```python
from build123d import *

# Parameters (mm, degrees)
SKETCH1_R           = 2.25
SKETCH1_W           = 40.1
SKETCH1_H           = 20.1
BOSS_EXTRUDE1_DEPTH = 3.175
FILLET1_R           = 80
FILLET2_R           = 8


with BuildPart() as part:
    # Sketch1 → Boss-Extrude1 (new body)
    with BuildSketch(Plane(origin=(0, 0, 0), x_dir=(1, 0, 0), z_dir=(0, 1, 0))):
        with BuildLine():
            Line((-70, 14), (-40, 14))
            Line((-40, 14), (-39.816062711, 70))
            Line((-39.816062711, 70), (-73.623466631, 79.058666579))
            ThreePointArc((-73.623466631, 79.058666579), (-83.522961568, 96.205094778), (-66.376533369, 106.104589715))
            Line((-66.376533369, 106.104589715), (0, 88.319051202))
            Line((0, 88.319051202), (66.376533369, 106.104589715))
            ThreePointArc((66.376533369, 106.104589715), (83.522961568, 96.205094778), (73.623466631, 79.058666579))
            Line((73.623466631, 79.058666579), (39.816062711, 70))
            Line((39.816062711, 70), (40, 14))
            Line((40, 14), (70, 14))
            ThreePointArc((70, 14), (84, 0), (70, -14))
            Line((70, -14), (40, -14))
            Line((40, -14), (39.816062711, -70))
            Line((39.816062711, -70), (73.623466631, -79.058666579))
            ThreePointArc((73.623466631, -79.058666579), (83.522961568, -96.205094778), (66.376533369, -106.104589715))
            Line((66.376533369, -106.104589715), (0, -88.319051202))
            Line((0, -88.319051202), (-66.376533369, -106.104589715))
            ThreePointArc((-66.376533369, -106.104589715), (-83.522961568, -96.205094778), (-73.623466631, -79.058666579))
            Line((-73.623466631, -79.058666579), (-39.816062711, -70))
            Line((-39.816062711, -70), (-40, -14))
            Line((-40, -14), (-70, -14))
            ThreePointArc((-70, -14), (-84, 0), (-70, 14))
        make_face()
        with Locations(Location((-76.433311385, 99.481809639, 0), (0, 0, 270))):
            Circle(SKETCH1_R, mode=Mode.SUBTRACT)
        with Locations(Location((-79.021501836, 89.822551376, 0), (0, 0, 270))):
            Circle(SKETCH1_R, mode=Mode.SUBTRACT)
        with Locations(Location((-78, 5, 0), (0, 0, 270))):
            Circle(SKETCH1_R, mode=Mode.SUBTRACT)
        with Locations(Location((-79.021501836, -89.822551376, 0), (0, 0, 90))):
            Circle(SKETCH1_R, mode=Mode.SUBTRACT)
        with Locations(Location((-76.433311385, -99.481809639, 0), (0, 0, 90))):
            Circle(SKETCH1_R, mode=Mode.SUBTRACT)
        with Locations(Location((-78, -5, 0), (0, 0, 270))):
            Circle(SKETCH1_R, mode=Mode.SUBTRACT)
        with Locations(Location((78, -5, 0), (0, 0, 90))):
            Circle(SKETCH1_R, mode=Mode.SUBTRACT)
        with Locations(Location((76.433311385, -99.481809639, 0), (0, 0, 270))):
            Circle(SKETCH1_R, mode=Mode.SUBTRACT)
        with Locations(Location((79.021501836, -89.822551376, 0), (0, 0, 270))):
            Circle(SKETCH1_R, mode=Mode.SUBTRACT)
        with Locations(Location((78, 5, 0), (0, 0, 90))):
            Circle(SKETCH1_R, mode=Mode.SUBTRACT)
        with Locations(Location((79.021501836, 89.822551376, 0), (0, 0, 90))):
            Circle(SKETCH1_R, mode=Mode.SUBTRACT)
        with Locations(Location((76.433311385, 99.481809639, 0), (0, 0, 90))):
            Circle(SKETCH1_R, mode=Mode.SUBTRACT)
        with Locations(Location((-30.95703272, 76.943715692, 0), (0, 0, 90))):
            Circle(SKETCH1_R, mode=Mode.SUBTRACT)
        with Locations(Location((-28.368842269, 86.602973955, 0), (0, 0, 90))):
            Circle(SKETCH1_R, mode=Mode.SUBTRACT)
        with Locations(Location((-28.24, -5, 0), (0, 0, 90))):
            Circle(SKETCH1_R, mode=Mode.SUBTRACT)
        with Locations(Location((-28.24, 5, 0), (0, 0, 90))):
            Circle(SKETCH1_R, mode=Mode.SUBTRACT)
        with Locations(Location((-28.368842269, -86.602973955, 0), (0, 0, 270))):
            Circle(SKETCH1_R, mode=Mode.SUBTRACT)
        with Locations(Location((-30.95703272, -76.943715692, 0), (0, 0, 270))):
            Circle(SKETCH1_R, mode=Mode.SUBTRACT)
        with Locations(Location((28.368842269, 86.602973955, 0), (0, 0, 270))):
            Circle(SKETCH1_R, mode=Mode.SUBTRACT)
        with Locations(Location((30.95703272, 76.943715692, 0), (0, 0, 270))):
            Circle(SKETCH1_R, mode=Mode.SUBTRACT)
        with Locations(Location((28.24, 5, 0), (0, 0, 270))):
            Circle(SKETCH1_R, mode=Mode.SUBTRACT)
        with Locations(Location((28.24, -5, 0), (0, 0, 270))):
            Circle(SKETCH1_R, mode=Mode.SUBTRACT)
        with Locations(Location((30.95703272, -76.943715692, 0), (0, 0, 90))):
            Circle(SKETCH1_R, mode=Mode.SUBTRACT)
        with Locations(Location((28.368842269, -86.602973955, 0), (0, 0, 90))):
            Circle(SKETCH1_R, mode=Mode.SUBTRACT)
        Polygon((-70.460853466, 103.109639074), (-75.663116273, 83.694529965), (-36.929490638, 73.315886257), (-31.727227832, 92.730995365), align=None, mode=Mode.SUBTRACT)
        with Locations((-53.12, 0)):
            Rectangle(SKETCH1_W, SKETCH1_H, mode=Mode.SUBTRACT)
        Polygon((-36.929490638, -73.315886257), (-31.727227832, -92.730995365), (-70.460853466, -103.109639074), (-75.663116273, -83.694529965), align=None, mode=Mode.SUBTRACT)
        Polygon((36.929490638, 73.315886257), (31.727227832, 92.730995365), (70.460853466, 103.109639074), (75.663116273, 83.694529965), align=None, mode=Mode.SUBTRACT)
        with Locations((53.12, 0)):
            Rectangle(SKETCH1_W, SKETCH1_H, mode=Mode.SUBTRACT)
        Polygon((36.929490638, -73.315886257), (31.727227832, -92.730995365), (70.460853466, -103.109639074), (75.663116273, -83.694529965), align=None, mode=Mode.SUBTRACT)
    extrude(amount=BOSS_EXTRUDE1_DEPTH)

    # Fillet1
    fillet1_edges = [part.edges().sort_by_distance(p)[0] for p in [
        (0, 1.5875, -88.319051202),
        (0, 1.5875, 88.319051202),
    ]]
    fillet(fillet1_edges, radius=FILLET1_R)

    # Fillet2
    fillet2_edges = [part.edges().sort_by_distance(p)[0] for p in [
        (-40, 1.5875, -14),
        (-39.816062711, 1.5875, -70),
        (39.816062711, 1.5875, -70),
        (40, 1.5875, -14),
        (40, 1.5875, 14),
        (39.816062711, 1.5875, 70),
        (-39.816062711, 1.5875, 70),
        (-40, 1.5875, 14),
    ]]
    fillet(fillet2_edges, radius=FILLET2_R)


solid = part.part
```
Here's how the part is built. I have some questions about the finished solid (model axes, mm). A direction names the side the tool comes from. Round coordinates to 2 decimals unless told otherwise and drop trailing zeros. Order: outer loops, then holes, each group sorted by start corner. A loop starts at its lowest first (then second) coordinate and runs counter-clockwise, first axis right, second up. Notation, with made-up numbers: (62, 14) -> (85, 14) arc R21 cw to (85, 32) -> close; hole circle Ø1 at (38, 73.5). An arc over 180 degrees is marked (long way). Use a Markdown table: item, result. Add a question column.
(1) If we mould it in two halves opening along X, with no side actions, what happens to faces 1 (the face through (-41.44, 1.61, 68.67)), 2 (the face through (41.44, 1.61, 68.67)), 3 (the face through (56.57, 1.57, 78.58))? For each: released by +X, released by -X, zero draft, split by the parting line, or undercut.
(2) I need wall thicknesses on line 1 along Z through (x, y) = (-45.5, 2); line 2 along Z through (x, y) = (-37, 2.8); line 3 along Z through (x, y) = (-27.5, 2.75). Which ranges of each line are inside material? Lowest first, please.
(3) Suppose I cut it at C-C, the plane y = 2.65. Count the separate pieces of the cut face and the enclosed holes in it, and give its area (3 significant figures).
(4) Suppose I cut it at B-B, the plane z = -5. Please give me the cut outline in (x, y) (3 decimals), and give its area (3 significant figures).
(5) Suppose I cut it at A-A, the plane x = -51. Please give me the cut outline in (y, z) (3 decimals), and give its area (3 significant figures).
(6) Suppose I cut it at D-D, the plane z = 60. Please give me the cut outline in (x, y) (3 decimals).
(7) For pin 1 Ø1 at (x, y) = (-61.5, 2.5) entering from +Z; pin 2 Ø1 at (y, z) = (1.5, 3) entering from +X (3 decimals); pin 3 Ø1 at (y, z) = (1.5, -3.5) entering from +X, each with a flat end and sliding along its axis, tell me the tip position at first contact or that it passes through.
(8) For faces 4 (the face through (-43.86, 1.57, -100.07)), 5 (the face through (34.365, 1.565, -82.888)), which set-ups out of +Z, -Z, +X, -X, +Y, -Y let a thin tool reach every point of the face, with its end or its side?
Verdict:
| question | item | result |
|---|---|---|
| 1 | face 1 | released by -X |
| 1 | face 2 | released by +X |
| 1 | face 3 | undercut |
| 2 | line 1 | -100.51 to -96.42, -75.61 to -71.52, -14.39 to -10.05, 10.05 to 14.39, 71.52 to 75.61, 96.42 to 100.51 |
| 2 | line 2 | -98.23 to -94.14, -73.33 to -10.05, 10.05 to 73.33, 94.14 to 98.23 |
| 2 | line 3 | -95.69 to -88.68, -84.53 to -7.12, -2.88 to 2.88, 7.12 to 84.53, 88.68 to 95.69 |
| 3 | separate pieces | 1 |
| 3 | enclosed holes | 30 |
| 3 | area | 16,900 mm2 |
| 4 | outline | (-83.077, 0) -> (-80.25, 0) -> (-80.25, 3.175) -> (-83.077, 3.175) -> close; (-75.75, 0) -> (-73.17, 0) -> (-73.17, 3.175) -> (-75.75, 3.175) -> close; (-33.07, 0) -> (-30.49, 0) -> (-30.49, 3.175) -> (-33.07, 3.175) -> close; (-25.99, 0) -> (25.99, 0) -> (25.99, 3.175) -> (-25.99, 3.175) -> close; (30.49, 0) -> (33.07, 0) -> (33.07, 3.175) -> (30.49, 3.175) -> close; (73.17, 0) -> (75.75, 0) -> (75.75, 3.175) -> (73.17, 3.175) -> close; (80.25, 0) -> (83.077, 0) -> (83.077, 3.175) -> (80.25, 3.175) -> close |
| 4 | area | 216 mm2 |
| 5 | outline | (0, -101.984) -> (3.175, -101.984) -> (3.175, -97.895) -> (0, -97.895) -> close; (0, -77.086) -> (3.175, -77.086) -> (3.175, -72.997) -> (0, -72.997) -> close; (0, -14) -> (3.175, -14) -> (3.175, -10.05) -> (0, -10.05) -> close; (0, 10.05) -> (3.175, 10.05) -> (3.175, 14) -> (0, 14) -> close; (0, 72.997) -> (3.175, 72.997) -> (3.175, 77.086) -> (0, 77.086) -> close; (0, 97.895) -> (3.175, 97.895) -> (3.175, 101.984) -> (0, 101.984) -> close |
| 5 | area | 77.0 mm2 |
| 6 | outline | (-39.849, 0) -> (39.849, 0) -> (39.849, 3.175) -> (-39.849, 3.175) -> close |
| 7 | pin 1 | z = 104.93 |
| 7 | pin 2 | x = 83.775 |
| 7 | pin 3 | x = 83.67 |
| 8 | face 4 | -Z, +Y, -Y |
| 8 | face 5 | +Y, -Y |
